Autodesk Inventor part; units mm, degrees
ref_plane "YZ Plane" through (0, 0, 0) normal (1, 0, 0) x (0, 1, 0)
ref_plane "XZ Plane" through (0, 0, 0) normal (0, 1, 0) x (-1, 0, 0)
ref_plane "XY Plane" through (0, 0, 0) normal (0, 0, 1) x (1, 0, 0)
sketch "Sketch1" plane through (0, 0, 0) normal (0, 1, 0) x (-1, 0, 0)
  line L0 (5, -2.5) -> (5, -47.5)
  line L1 (0, -47.5) -> (0, -2.5)
  arc A0 (5, -2.5) -> (0, -2.5) centre (2.5, -2.5) ccw
  arc A1 (0, -47.5) -> (5, -47.5) centre (2.5, -47.5) ccw
  circle A2 centre (2.5, -2.5) radius 1.5
  circle A3 centre (2.5, -47.5) radius 1.5
  point P0 (0, 0)
  dimension "d2" = 3
  dimension "d3" = 3
extrude "Extrusion1" add sketch "Sketch1" along normal blind 5
properties part number "gripper1"
Design review of the part built by this model. Coordinates are the model's own, in mm. Coordinates: 2 decimals unless noted, no trailing zeros. Loops run counter-clockwise (first coordinate to the right, second up) from the corner with the lowest first, then second, coordinate; pieces in that order, holes last. Notation, with made-up numbers: (-12, -18.5) - (47, -18.5) arc R21 cw to (47, 15.5) - close; hole circle Ø9 at (51, 23.5). An arc over 180 degrees is marked (long way). Use CSV: the item, a comma, the result in double quotes. Start each with the question number.
1. Add section A-A on x = -2.5. Give the boundary of the cut face in (y, z), plus the area to 3 significant figures.
2. Mouldability with a two-part tool opening along X and no side actions: class faces 1 (the cylindrical face through (-2.175, 2.465, -46.036)), 2 (the flat face through (0, 2, -25)), 3 (the cylindrical face through (-2.4, 2.5, 0)) as released by +X, released by -X, zero draft, split by the parting line, or undercut.
3. Add section B-B on y = 2.3. Give the boundary of the cut face in (x, z).
4. Add section C-C on x = -4.45. Give the boundary of the cut face in (y, z).
5. Clearance check with a flat-ended pin moving along its axis: pin 1 (1.8 mm diameter, centred on x = -2.5, z = -2.5, fed in from +Y). State where the tip first meets the part, or that it passes through.
6. To check wall thickness, follow probe 1 along Z at (x, y) = (-2.5, 2.2); probe 2 along Z at (x, y) = (-1.45, 0.8); probe 3 along X at (y, z) = (4.7, -48). State the ranges of each line that lie inside material, in increasing order.
Resolved:
1,outline,"(0, -50) - (5, -50) - (5, -49) - (0, -49) - close; (0, -46) - (5, -46) - (5, -4) - (0, -4) - close; (0, -1) - (5, -1) - (5, 0) - (0, 0) - close"
1,area,"220 mm2"
2,face 1,"undercut"
2,face 2,"released by +X"
2,face 3,"split by the parting line"
3,outline,"(-5, -47.5) arc R2.5 ccw to (0, -47.5) - (0, -2.5) arc R2.5 ccw to (-5, -2.5) - close; hole circle Ø3 at (-2.5, -47.5); hole circle Ø3 at (-2.5, -2.5)"
4,outline,"(0, -49.06) - (5, -49.06) - (5, -0.94) - (0, -0.94) - close"
5,pin 1,"through"
6,probe 1,"-50 to -49, -46 to -4, -1 to 0"
6,probe 2,"-49.77 to -48.57, -46.43 to -3.57, -1.43 to -0.23"
6,probe 3,"-4.95 to -3.91, -1.09 to -0.05"
